```python
from build123d import *

# Parameters (mm, degrees)
SKETCH1_R           = 50
SKETCH1_W           = 60
SKETCH1_H           = 40
SKETCH1_W_2         = 45
SKETCH1_H_2         = 24.4
BOSS_EXTRUDE1_DEPTH = 5
CUT_EXTRUDE1_REACH  = 7
SKETCH8_R           = 1.025
SKETCH9_R           = 50
BOSS_EXTRUDE2_DEPTH = 32.75
SKETCH10_R          = 45
CUT_EXTRUDE2_DEPTH  = 32.75
SKETCH11_R          = 50
BOSS_EXTRUDE3_DEPTH = 2.75
SKETCH12_R          = 11
CUT_EXTRUDE3_DEPTH  = 2.75


with BuildPart() as part:
    # Sketch1 → Boss-Extrude1 (new body)
    with BuildSketch(Plane(origin=(0, 0, 0), x_dir=(1, 0, 0), z_dir=(0, 1, 0))):
        with Locations((17, 20)):
            Circle(SKETCH1_R)
        with Locations((30, 20)):
            Rectangle(SKETCH1_W, SKETCH1_H, mode=Mode.SUBTRACT)
        with Locations((30, 20)):
            Rectangle(SKETCH1_W, SKETCH1_H)
        with Locations((27.5, 20)):
            Rectangle(SKETCH1_W_2, SKETCH1_H_2, mode=Mode.SUBTRACT)
    extrude(amount=BOSS_EXTRUDE1_DEPTH)

    # Sketch8 → Cut-Extrude1 (cut, up to next)
    with BuildSketch(Plane(origin=(0, 0, 0), x_dir=(-1, 0, 0), z_dir=(0, -1, 0)), mode=Mode.PRIVATE) as cut_extrude1_sk1:
        with Locations((-52.8, 28.5)):
            Circle(SKETCH8_R)
    cut_extrude1_tool1 = extrude(cut_extrude1_sk1.sketch, amount=-CUT_EXTRUDE1_REACH, mode=Mode.PRIVATE) & part.part
    add(cut_extrude1_tool1.solids().sort_by_distance((52.8, 0, -28.5))[0], mode=Mode.SUBTRACT)
    # Sketch8 → Cut-Extrude1 (cut, up to next)
    with BuildSketch(Plane(origin=(0, 0, 0), x_dir=(-1, 0, 0), z_dir=(0, -1, 0)), mode=Mode.PRIVATE) as cut_extrude1_sk2:
        with Locations((-46.5, 35)):
            Circle(SKETCH8_R)
    cut_extrude1_tool2 = extrude(cut_extrude1_sk2.sketch, amount=-CUT_EXTRUDE1_REACH, mode=Mode.PRIVATE) & part.part
    add(cut_extrude1_tool2.solids().sort_by_distance((46.5, 0, -35))[0], mode=Mode.SUBTRACT)
    # Sketch8 → Cut-Extrude1 (cut, up to next)
    with BuildSketch(Plane(origin=(0, 0, 0), x_dir=(-1, 0, 0), z_dir=(0, -1, 0)), mode=Mode.PRIVATE) as cut_extrude1_sk3:
        with Locations((-29.5, 35)):
            Circle(SKETCH8_R)
    cut_extrude1_tool3 = extrude(cut_extrude1_sk3.sketch, amount=-CUT_EXTRUDE1_REACH, mode=Mode.PRIVATE) & part.part
    add(cut_extrude1_tool3.solids().sort_by_distance((29.5, 0, -35))[0], mode=Mode.SUBTRACT)
    # Sketch8 → Cut-Extrude1 (cut, up to next)
    with BuildSketch(Plane(origin=(0, 0, 0), x_dir=(-1, 0, 0), z_dir=(0, -1, 0)), mode=Mode.PRIVATE) as cut_extrude1_sk4:
        with Locations((-12.5, 35)):
            Circle(SKETCH8_R)
    cut_extrude1_tool4 = extrude(cut_extrude1_sk4.sketch, amount=-CUT_EXTRUDE1_REACH, mode=Mode.PRIVATE) & part.part
    add(cut_extrude1_tool4.solids().sort_by_distance((12.5, 0, -35))[0], mode=Mode.SUBTRACT)
    # Sketch8 → Cut-Extrude1 (cut, up to next)
    with BuildSketch(Plane(origin=(0, 0, 0), x_dir=(-1, 0, 0), z_dir=(0, -1, 0)), mode=Mode.PRIVATE) as cut_extrude1_sk5:
        with Locations((-12.5, 5)):
            Circle(SKETCH8_R)
    cut_extrude1_tool5 = extrude(cut_extrude1_sk5.sketch, amount=-CUT_EXTRUDE1_REACH, mode=Mode.PRIVATE) & part.part
    add(cut_extrude1_tool5.solids().sort_by_distance((12.5, 0, -5))[0], mode=Mode.SUBTRACT)
    # Sketch8 → Cut-Extrude1 (cut, up to next)
    with BuildSketch(Plane(origin=(0, 0, 0), x_dir=(-1, 0, 0), z_dir=(0, -1, 0)), mode=Mode.PRIVATE) as cut_extrude1_sk6:
        with Locations((-29.5, 5)):
            Circle(SKETCH8_R)
    cut_extrude1_tool6 = extrude(cut_extrude1_sk6.sketch, amount=-CUT_EXTRUDE1_REACH, mode=Mode.PRIVATE) & part.part
    add(cut_extrude1_tool6.solids().sort_by_distance((29.5, 0, -5))[0], mode=Mode.SUBTRACT)
    # Sketch8 → Cut-Extrude1 (cut, up to next)
    with BuildSketch(Plane(origin=(0, 0, 0), x_dir=(-1, 0, 0), z_dir=(0, -1, 0)), mode=Mode.PRIVATE) as cut_extrude1_sk7:
        with Locations((-46.5, 5)):
            Circle(SKETCH8_R)
    cut_extrude1_tool7 = extrude(cut_extrude1_sk7.sketch, amount=-CUT_EXTRUDE1_REACH, mode=Mode.PRIVATE) & part.part
    add(cut_extrude1_tool7.solids().sort_by_distance((46.5, 0, -5))[0], mode=Mode.SUBTRACT)
    # Sketch8 → Cut-Extrude1 (cut, up to next)
    with BuildSketch(Plane(origin=(0, 0, 0), x_dir=(-1, 0, 0), z_dir=(0, -1, 0)), mode=Mode.PRIVATE) as cut_extrude1_sk8:
        with Locations((-52.8, 11.5)):
            Circle(SKETCH8_R)
    cut_extrude1_tool8 = extrude(cut_extrude1_sk8.sketch, amount=-CUT_EXTRUDE1_REACH, mode=Mode.PRIVATE) & part.part
    add(cut_extrude1_tool8.solids().sort_by_distance((52.8, 0, -11.5))[0], mode=Mode.SUBTRACT)

    # Sketch9 → Boss-Extrude2 (add)
    with BuildSketch(Plane(origin=(0, 5, 0), x_dir=(1, 0, 0), z_dir=(0, 1, 0))):
        with Locations((17, 20)):
            Circle(SKETCH9_R)
    extrude(amount=BOSS_EXTRUDE2_DEPTH)

    # Sketch10 → Cut-Extrude2 (cut)
    with BuildSketch(Plane(origin=(0, 37.75, 0), x_dir=(1, 0, 0), z_dir=(0, 1, 0))):
        with Locations((17, 20)):
            Circle(SKETCH10_R)
    extrude(amount=-CUT_EXTRUDE2_DEPTH, mode=Mode.SUBTRACT)

    # Sketch11 → Boss-Extrude3 (add)
    with BuildSketch(Plane(origin=(0, 37.75, 0), x_dir=(1, 0, 0), z_dir=(0, 1, 0))):
        with Locations((17, 20)):
            Circle(SKETCH11_R)
    extrude(amount=BOSS_EXTRUDE3_DEPTH)

    # Sketch12 → Cut-Extrude3 (cut)
    with BuildSketch(Plane(origin=(0, 40.5, 0), x_dir=(1, 0, 0), z_dir=(0, 1, 0))):
        with Locations((17, 20)):
            Circle(SKETCH12_R)
    extrude(amount=-CUT_EXTRUDE3_DEPTH, mode=Mode.SUBTRACT)


solid = part.part
```
Input: part model. Units: mm. Frame: model coordinates. A direction names the side the tool comes from. Round coordinates to 2 decimals unless told otherwise and drop trailing zeros. Write each loop counter-clockwise with the first axis right and the second up, starting at its lowest first coordinate (ties: lowest second). Pieces come first, ordered by that corner, then holes. Notation, with made-up numbers: (31, 44.25) - (42, 44.25) arc R19 cw to (42, 49.25) - close; hole circle Ø10 at (12.25, 82). An arc over 180 degrees is marked (long way). Write item = value, one per line.
(1) Pull-direction query (Z, two-part tool) for faces 4 (the flat face through (16, 40.5, -32)), 5 (the cylindrical face through (64.69, 19.97, -35.02)), 6 (the flat face through (27, 2, -7.8)), 7 (the cylindrical face through (22.076, 39.144, -10.241)); classes: +Z half, -Z half, draft (parallel to the pull), parting line (faces both ways), or undercut.
Geometry check:
face_4 = draft
face_5 = parting line
face_6 = undercut
face_7 = undercut
(2) Section query A-A on x = 17. Output: boundary loops of the cut face in (y, z).
Geometry check:
outline = (0, -70) - (40.5, -70) - (40.5, -31) - (37.75, -31) - (37.75, -65) - (5, -65) - (5, -32.2) - (0, -32.2) - close; (0, -7.8) - (5, -7.8) - (5, 25) - (37.75, 25) - (37.75, -9) - (40.5, -9) - (40.5, 30) - (0, 30) - close
(3) Material intervals for probe 1 along Z at (x, y) = (46.5, 1.9) (3 decimals); probe 2 along Z at (x, y) = (16, 33); probe 3 along Y at (x, z) = (-17, -46), sorted ascending.
Geometry check:
probe_1 = -60.37 to -36.025, -33.975 to -32.2, -7.8 to -6.025, -3.975 to 20.37
probe_2 = -69.99 to -64.99, 24.99 to 29.99
probe_3 = 0 to 5, 37.75 to 40.5
(4) Section query D-D on x = 58.5. Output: boundary loops of the cut face in (y, z).
Geometry check:
outline = (0, -47.89) - (40.5, -47.89) - (40.5, 7.89) - (0, 7.89) - close; hole (5, -37.4) - (37.75, -37.4) - (37.75, -2.6) - (5, -2.6) - close
(5) Section query C-C on z = 14. Output: boundary loops of the cut face in (x, y), then the cut area to 3 significant figures.
Geometry check:
outline = (-19.66, 0) - (53.66, 0) - (53.66, 40.5) - (-19.66, 40.5) - close; hole (-12.48, 5) - (46.48, 5) - (46.48, 37.75) - (-12.48, 37.75) - close
area = 1,040 mm^2
(6) Contact query for flat-ended pins moving along their axis: pin 1 Ø1.5 at (x, y) = (32.5, 2.5) entering from -Z; pin 2 Ø6 at (x, y) = (29, 15) entering from -Z; pin 3 Ø2.5 at (y, z) = (2.5, -18) entering from -X. Output: stop coordinate, or through.
Geometry check:
pin_1 = -67.77
pin_2 = -69.18
pin_3 = -32.99
(7) Access query for faces 1 (the flat face through (16, 5, -1)), 2 (the flat face through (50, 2, -20)), 3 (the flat face through (16, 0, 2)). Directions: +Z, -Z, +X, -X, +Y, -Y. A direction counts if a zero-diameter tool reaches every point of the face in a straight line with its end or side. Return the directions, or none.
Geometry check:
face_1 = none
face_2 = -Y
face_3 = +Z, -Z, +X, -X, -Y
(8) Section query B-B on z = -20. Output: boundary loops of the cut face in (x, y).
Geometry check:
outline = (-33, 0) - (5, 0) - (5, 5) - (-28, 5) - (-28, 37.75) - (6, 37.75) - (6, 40.5) - (-33, 40.5) - close; (28, 37.75) - (62, 37.75) - (62, 5) - (50, 5) - (50, 0) - (67, 0) - (67, 40.5) - (28, 40.5) - close
